For this review, use the dimensioned drawing (mm, ordinates from the lowest corner) and the shaded views. Give positions to 0.01 mm unless a question says otherwise; leave off trailing zeros. Write each loop counter-clockwise with the first axis right and the second up, starting at its lowest first coordinate (ties: lowest second). Pieces come first, ordered by that corner, then holes. Notation, with made-up numbers: (14.5, 48) -> (27.5, 48) arc R16 ccw to (27.5, 59) -> close; hole circle Ø6 at (8, 62.5). An arc over 180 degrees is marked (long way). Write each question's results on one line, items separated by ' | '. Start each with the question number.
(1) To check wall thickness, follow probe 1 along X at (y, z) = (1.65, 32); probe 2 along X at (y, z) = (1.3, 2.5); probe 3 along Z at (x, y) = (16.5, 3.1). State the ranges of each line that lie inside material, in increasing order.
(2) Clearance check with flat-ended pins moving along their axes: pin 1 (3 mm diameter, centred on x = 108, y = 4, fed in from +Z); pin 2 (3 mm diameter, centred on x = 90.5, y = 5, fed in from -Z); pin 3 (1.8 mm diameter, centred on y = 3.5, z = 2.5, fed in from +X). State where each tip first meets the part, or that it passes through.
(3) Take a section at A-A (z = 2). State the section outline as (x, y) points.
(4) Take a section at B-B (y = 1.3). State the section outline as (x, z) points.
(5) Take a section at C-C (x = 42.5). State the section outline as (y, z) points.
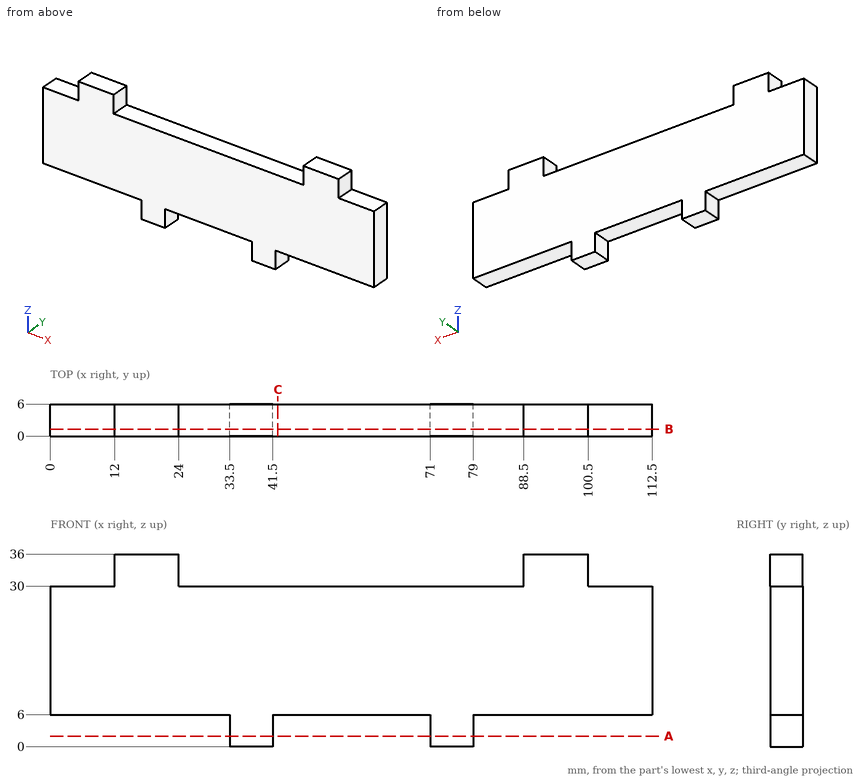
Report:
1) probe 1: 12 to 24, 88.5 to 100.5 | probe 2: 33.5 to 41.5, 71 to 79 | probe 3: 6 to 36
2) pin 1: z = 30 | pin 2: z = 6 | pin 3: x = 79
3) outline: (33.5, 0) -> (41.5, 0) -> (41.5, 6) -> (33.5, 6) -> close; (71, 0) -> (79, 0) -> (79, 6) -> (71, 6) -> close
4) outline: (0, 6) -> (33.5, 6) -> (33.5, 0) -> (41.5, 0) -> (41.5, 6) -> (71, 6) -> (71, 0) -> (79, 0) -> (79, 6) -> (112.5, 6) -> (112.5, 30) -> (100.5, 30) -> (100.5, 36) -> (88.5, 36) -> (88.5, 30) -> (24, 30) -> (24, 36) -> (12, 36) -> (12, 30) -> (0, 30) -> close
5) outline: (0, 6) -> (6, 6) -> (6, 30) -> (0, 30) -> close
